The listing builds one solid part. Answer for the finished solid, in the listing's coordinates (mm). Give positions to 0.01 mm unless a question says otherwise; leave off trailing zeros. Write each loop counter-clockwise with the first axis right and the second up, starting at its lowest first coordinate (ties: lowest second). Pieces come first, ordered by that corner, then holes. Notation, with made-up numbers: (49.25, -1.5) -> (68.25, -1.5) arc R19 cw to (68.25, 13.5) -> close; hole circle Ø9 at (61.5, 81.25). An arc over 180 degrees is marked (long way). One line per question, with ' | ' between items.
from build123d import *

# Parameters (mm, degrees)
SKETCH1_R           = 4.7625
BOSS_EXTRUDE1_DEPTH = 2.38125
SKETCH4_R           = 1.6764
SKETCH4_R_2         = 2.38125
CUT_EXTRUDE2_DEPTH  = 269.420180625
SKETCH5_R           = 1.6764
CUT_EXTRUDE3_DEPTH  = 269.420180625
SKETCH6_R           = 3.175
CUT_EXTRUDE4_DEPTH  = 269.420180625


with BuildPart() as part:
    # Sketch1 → Boss-Extrude1 (new body)
    with BuildSketch(Plane.XY):
        Polygon((0, 0), (25.4, 43.994090512), (82.55, 43.994090512), (82.55, 59.869090512), (16.234564477, 59.869090512), (-9.165435523, 15.875), (-217.739113558, 15.875), (-241.968881923, 78.201036741), (-256.765108354, 72.448879893), (-228.6, 0), align=None)
        with Locations(Location((-58.42, 7.9375, 0), (0, 0, 180))):
            Circle(SKETCH1_R, mode=Mode.SUBTRACT)
    extrude(amount=BOSS_EXTRUDE1_DEPTH)

    # Sketch4 → Cut-Extrude2 (cut, through all)
    with BuildSketch(Plane.XY.offset(2.38125)):
        with Locations((74.93, 51.931590512)):
            Circle(SKETCH4_R)
        with Locations((-246.937589356, 69.075817516)):
            Circle(SKETCH4_R_2)
    extrude(amount=-CUT_EXTRUDE2_DEPTH, mode=Mode.SUBTRACT)

    # Sketch5 → Cut-Extrude3 (cut, through all)
    with BuildSketch(Plane.XY.offset(2.38125)):
        with Locations((-147.32, 7.9375)):
            Circle(SKETCH5_R)
        with Locations((-121.92, 7.9375)):
            Circle(SKETCH5_R)
        with Locations((-224.653180894, 11.753814283)):
            Circle(SKETCH5_R)
        with Locations((-233.856631852, 35.427776572)):
            Circle(SKETCH5_R)
    extrude(amount=-CUT_EXTRUDE3_DEPTH, mode=Mode.SUBTRACT)

    # Sketch6 → Cut-Extrude4 (cut, through all)
    with BuildSketch(Plane.XY.offset(2.38125)):
        with Locations((-214.564113558, 7.9375)):
            Circle(SKETCH6_R)
    extrude(amount=-CUT_EXTRUDE4_DEPTH, mode=Mode.SUBTRACT)


solid = part.part
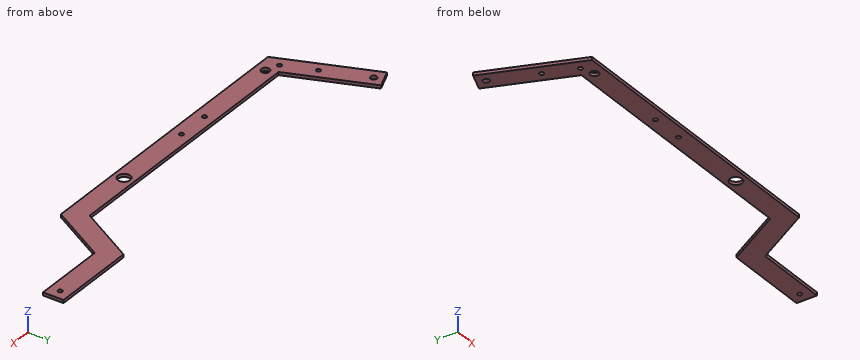
Item 1: Consider line 1 (Y direction, x = -121.92, z = 1.75) (3 decimals); line 2 (X direction, y = 8, z = 2.05); line 3 (Y direction, x = 74.93, z = 1.7). Determine where each line is inside the solid, lowest interval first. Write a range as [from, to].
Answers below:
line 1: [0, 6.261], [9.614, 15.875] | line 2: [-231.71, -217.74], [-211.39, -149], [-145.64, -123.6], [-120.24, -63.18], [-53.66, 4.62] | line 3: [43.99, 50.26], [53.61, 59.87]
Item 2: Flat-ended cylindrical pins translate along their axes: pin 1 (3 mm diameter, centred on x = -147.32, y = 7.94, fed in from +Z); pin 2 (1.2 mm diameter, centred on x = 37.5, z = 0.5, fed in from +Y). Find the tip coordinate at first contact, or state that the pin passes through.
Answers below:
pin 1: through | pin 2: y = 59.87
Item 3: Find section A-A (x = -58.42). Write down the section's boundary in (y, z) (3 decimals).
Answers below:
outline: (0, 0) -> (3.175, 0) -> (3.175, 2.381) -> (0, 2.381) -> close; (12.7, 0) -> (15.875, 0) -> (15.875, 2.381) -> (12.7, 2.381) -> close
Item 4: Find section B-B (z = 0.8). Count the separate pieces of the cut face and the enclosed holes in it, then the cut area to 3 significant figures.
Answers below:
separate pieces: 1 | enclosed holes: 8 | area: 6,240 mm²
Item 5: Find section C-C (x = -138.5). Write down the section's boundary in (y, z) (3 decimals).
Answers below:
outline: (0, 0) -> (15.875, 0) -> (15.875, 2.381) -> (0, 2.381) -> close
